Part model, mm, in its own coordinate system. A direction names the side the tool comes from. Round coordinates to 2 decimals unless told otherwise and drop trailing zeros. Loops run counter-clockwise (first coordinate to the right, second up) from the corner with the lowest first, then second, coordinate; pieces in that order, holes last. Notation, with made-up numbers: M -12,20.5 L -4,20.5 A25 cw -4,51.5 Z; hole C 9.25,77.25 d2. An arc over 180 degrees is marked long. Put each result on its own line as item: value. Start each with the question number.
```python
from build123d import *

# Parameters (mm, degrees)
TORUS_R               = 6
TORUS_ANGLE           = 100
TORUS_PLACEMENT_ANGLE = 140
CYLINDER002_R         = 8
CYLINDER002_DEPTH     = 10
CYLINDER001_R         = 8
CYLINDER001_DEPTH     = 10
CYLINDER_R            = 40
CYLINDER_DEPTH        = 4


with BuildPart() as torus:
    # Torus → Torus (revolve)
    with BuildSketch(Plane.XZ):
        with Locations((30, 0)):
            Circle(TORUS_R)
    revolve(axis=Axis((0, 0, 0), (0, 0, 1)), revolution_arc=TORUS_ANGLE)


with BuildPart() as torus_1:
    # Torus placement: moved
    add(torus.part.moved(Location((0, 2, 7))).rotate(Axis((0, 2, 7), (0, 0, -1)), TORUS_PLACEMENT_ANGLE))


with BuildPart() as cylinder002:
    # Cylinder002 → Cylinder002 (new body)
    with BuildSketch(Plane(origin=(15, 10, 1), x_dir=(1, 0, 0), z_dir=(0, 0, 1))):
        Circle(CYLINDER002_R)
    extrude(amount=CYLINDER002_DEPTH)


with BuildPart() as cylinder001:
    # Cylinder001 → Cylinder001 (new body)
    with BuildSketch(Plane(origin=(-15, 10, 1), x_dir=(1, 0, 0), z_dir=(0, 0, 1))):
        Circle(CYLINDER001_R)
    extrude(amount=CYLINDER001_DEPTH)


with BuildPart() as cut002:
    # Cylinder → Cylinder (new body)
    with BuildSketch(Plane.XY):
        Circle(CYLINDER_R)
    extrude(amount=CYLINDER_DEPTH)

    # Cut: cut Cylinder001
    add(cylinder001.part, mode=Mode.SUBTRACT)

    # Cut001: cut Cylinder002
    add(cylinder002.part, mode=Mode.SUBTRACT)

    # Cut002: cut Torus
    add(torus_1.part, mode=Mode.SUBTRACT)


solid = cut002.part
```
1. Mould opens along X. For faces 3 (the flat face through (-22.93, -17.24, 2.85)), 4 (the flat face through (-1, 1, 4)), 5 (the cylindrical face through (-8.67, -39.05, 1.97)) say: released by +X, released by -X, zero draft, split by the parting line, or undercut.
2. Cut at A-A, the plane z = 1.95. Give the cut face in (x, y), and give its area (3 significant figures).
3. Wall check: L1, parallel to Y at x = -15, z = 1.7; L2, parallel to Y at x = -15, z = 2.7; L3, parallel to X at y = 5, z = 1.15 (3 decimals). Give the ranges that are in metal, low to high.
4. Cut at D-D, the plane y = 26.5. Give the cut face in (x, z), and give its area (3 significant figures).
5. Cut at C-C, the plane x = 0. Give the cut face in (y, z), and give its area (3 significant figures).
6. Drop flat-ended pins along their axis: pin 1 (8 mm diameter, centred on x = -14, y = 7, fed in from +Z); pin 2 (2 mm diameter, centred on y = 6, z = 2, fed in from -X); pin 3 (2 mm diameter, centred on y = -15.5, z = 2, fed in from +X). Give the stop position or say it passes through.
7. Which spindle directions (+Z, -Z, +X, -X, +Y, -Y) get a long thin tool onto all of the face, cutting with end or side? Do faces 1 (the flat face through (-1, 1, 0)), 2 (the flat face through (15, 10, 1)). Say none if no direction does.
8. Cut at B-B, the plane y = 10. Give the cut face in (x, z).
Results list:
1. face 3: undercut
1. face 4: zero draft
1. face 5: split by the parting line
2. outline: C 0,0 d80; hole M -25.46,-19.37 A33.24 ccw 25.46,-19.37 L 20.5,-15.2 A26.76 cw -20.5,-15.2 Z; hole C -15,10 d16; hole C 15,10 d16
2. area: 4,290 mm^2
3. L1: y = -37.08 to -27.18, -20.68 to 2, 18 to 37.08
3. L2: y = -37.08 to -28.72, -19.01 to 2, 18 to 37.08
3. L3: x = -39.686 to -21.245, -8.755 to 8.755, 21.245 to 39.686
4. outline: M -29.96,0 L 29.96,0 L 29.96,4 L -29.96,4 Z
4. area: 240 mm^2
5. outline: M -40,0 L 40,0 L 40,4 L -22.8,4 A6 cw -33.2,4 L -40,4 Z
5. area: 298 mm^2
6. pin 1: stops at z = 1
6. pin 2: stops at x = -39.69
6. pin 3: stops at x = 37.28
7. face 1: -Z, +X, -X, +Y, -Y
7. face 2: +Z
8. outline: M -38.73,0 L 38.73,0 L 38.73,4 L 23,4 L 23,1 L 7,1 L 7,4 L -7,4 L -7,1 L -23,1 L -23,4 L -38.73,4 Z
